```python
from build123d import *

# Parameters (mm, degrees)
ENL_V_MAT_EXTRU_1_DEPTH = 149.219431924
ESQUISSE3_R             = 3.75
ENL_V_MAT_EXTRU_2_DEPTH = 131.858702424
ENL_V_MAT_EXTRU_3_DEPTH = 126.862394907


with BuildPart() as part:
    # Esquisse1 → Révolution1 (revolve)
    with BuildSketch(Plane.XY, mode=Mode.PRIVATE) as r_volution1_sk:
        with BuildLine():
            Line((0, 0), (24.566275292, 0))
            Line((24.566275292, 0), (24.566275292, 25))
            Line((24.566275292, 25), (7.566275292, 25))
            ThreePointArc((7.566275292, 25), (6.152061729, 25.585786438), (5.566275292, 27))
            Line((5.566275292, 27), (5.566275292, 40))
            Line((5.566275292, 40), (-22.933724708, 40))
            Line((-22.933724708, 40), (-25.433724708, 37.5))
            Line((-25.433724708, 37.5), (-62.433724708, 37.5))
            Line((-62.433724708, 37.5), (-64.933724708, 40))
            Line((-64.933724708, 40), (-93.433724708, 40))
            Line((-93.433724708, 40), (-93.433724708, 27))
            ThreePointArc((-93.433724708, 27), (-94.019511146, 25.585786438), (-95.433724708, 25))
            Line((-95.433724708, 25), (-112.433724708, 25))
            Line((-112.433724708, 25), (-112.433724708, 0))
            Line((-112.433724708, 0), (0, 0))
        make_face()
    revolve(r_volution1_sk.sketch.rotate(Axis((-130.768922499, 0, 0), (1, 0, 0)), 90), axis=Axis((-130.768922499, 0, 0), (1, 0, 0)))

    # Esquisse2 → Enlèv. mat.-Extru.1 (cut, through all)
    with BuildSketch(Plane.ZY.offset(112.433724708)):
        with BuildLine():
            Line((0, 7), (0, 0))
            Line((0, 0), (43.449782835, 0))
            Line((43.449782835, 0), (43.449782835, 44.497429883))
            Line((43.449782835, 44.497429883), (0, 44.497429883))
            Line((0, 44.497429883), (0, 13))
            ThreePointArc((0, 13), (3, 10), (0, 7))
        make_face()
        with BuildLine():
            Line((-12, 7), (0, 7))
            ThreePointArc((0, 7), (3, 10), (0, 13))
            Line((0, 13), (-12, 13))
            ThreePointArc((-12, 13), (-15, 10), (-12, 7))
        make_face()
    extrude(amount=-ENL_V_MAT_EXTRU_1_DEPTH, mode=Mode.SUBTRACT)

    # Esquisse3 → Enlèv. mat.-Extru.2 (cut, through all)
    with BuildSketch(Plane.ZY.offset(93.433724708)):
        with Locations((-8.282209443, 30.909626441)):
            Circle(ESQUISSE3_R)
        with Locations((-22.627416998, 22.627416998)):
            Circle(ESQUISSE3_R)
        with Locations((-30.909626441, 8.282209443)):
            Circle(ESQUISSE3_R)
        with Locations((-30.909626441, -8.282209443)):
            Circle(ESQUISSE3_R)
        with Locations((-22.627416998, -22.627416998)):
            Circle(ESQUISSE3_R)
        with Locations((-8.282209443, -30.909626441)):
            Circle(ESQUISSE3_R)
        with Locations((8.282209443, -30.909626441)):
            Circle(ESQUISSE3_R)
        with Locations((22.627416998, -22.627416998)):
            Circle(ESQUISSE3_R)
        with Locations((30.909626441, -8.282209443)):
            Circle(ESQUISSE3_R)
    extrude(amount=-ENL_V_MAT_EXTRU_2_DEPTH, mode=Mode.SUBTRACT)

    # Esquisse4 → Enlèv. mat.-Extru.3 (cut, through all)
    with BuildSketch(Plane(origin=(0, 0, 0), x_dir=(1, 0, 0), z_dir=(0, 1, 0))):
        with BuildLine():
            Line((5.566275292, -31.140154495), (24.566275292, -40))
            Line((24.566275292, -40), (21.921370581, -25))
            Line((21.921370581, -25), (7.566275292, -25))
            ThreePointArc((7.566275292, -25), (6.152061729, -25.585786438), (5.566275292, -27))
            Line((5.566275292, -27), (5.566275292, -31.140154495))
        make_face()
        with BuildLine():
            Line((-5.433724708, -40), (5.566275292, -40))
            Line((5.566275292, -40), (5.566275292, -31.140154495))
            Line((5.566275292, -31.140154495), (-2.622958319, -27.321452148))
            ThreePointArc((-2.622958319, -27.321452148), (-4.722604922, -33.506811582), (-5.433724708, -40))
        make_face()
        with BuildLine():
            Line((-2.622958319, -27.321452148), (5.566275292, -31.140154495))
            Line((5.566275292, -31.140154495), (5.566275292, -27))
            ThreePointArc((5.566275292, -27), (6.152061729, -25.585786438), (7.566275292, -25))
            Line((7.566275292, -25), (21.921370581, -25))
            Line((21.921370581, -25), (19.356829962, -10.45576741))
            ThreePointArc((19.356829962, -10.45576741), (6.303432421, -16.199399791), (-2.622958319, -27.321452148))
        make_face()
        Polygon((5.566275292, -40), (24.566275292, -40), (5.566275292, -31.140154495), align=None)
        with BuildLine():
            Line((-7.154497255, -25.208360839), (-2.622958319, -27.321452148))
            ThreePointArc((-2.622958319, -27.321452148), (6.303432421, -16.199399791), (19.356829962, -10.45576741))
            Line((19.356829962, -10.45576741), (18.488589073, -5.531728645))
            ThreePointArc((18.488589073, -5.531728645), (3.259625276, -12.23263309), (-7.154497255, -25.208360839))
        make_face()
        with BuildLine():
            Line((21.921370581, -25), (24.566275292, -25))
            Line((24.566275292, -25), (24.566275292, -10))
            ThreePointArc((24.566275292, -10), (21.951603009, -10.114159057), (19.356829962, -10.45576741))
            Line((19.356829962, -10.45576741), (21.921370581, -25))
        make_face()
        Polygon((21.921370581, -25), (24.566275292, -40), (24.566275292, -25), align=None)
    extrude(amount=-ENL_V_MAT_EXTRU_3_DEPTH, mode=Mode.SUBTRACT)


solid = part.part
```
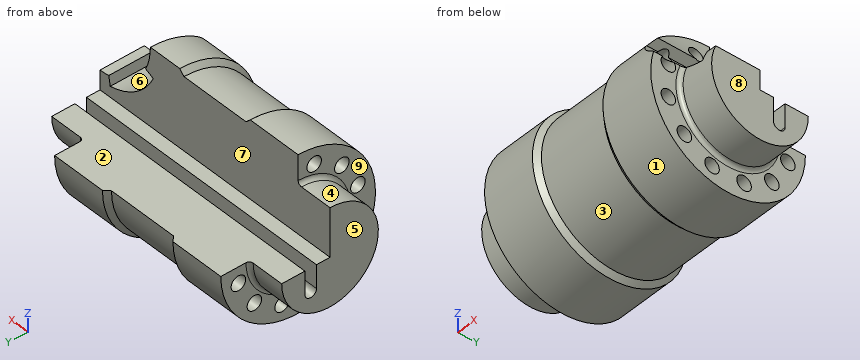
Geometry check sheet. Reference: the model listing, model coordinates, mm. Face numbers are marked on the shaded views. A direction names the side the tool comes from. Round coordinates to 2 decimals unless told otherwise and drop trailing zeros. Loops run counter-clockwise (first coordinate to the right, second up) from the corner with the lowest first, then second, coordinate; pieces in that order, holes last. Notation, with made-up numbers: (13, 28) - (37, 28) arc R21 ccw to (37, 54) - close; hole circle Ø8 at (26.5, 86). An arc over 180 degrees is marked (long way). Write each question's results on one line, items separated by ' | '. Start each with the question number.
Q1. Gauge pin test, flat ends, axial feed: P1, Ø2, axis at x = -66.5, y = 5, coming from the +Z side; P2, Ø3, axis at x = -75.5, z = -26.5, coming from the -Y side (3 decimals); P3, Ø1.5, axis at x = -92.5, z = 19, coming from the +Y side. Record the tip position at first contact, or that the pin passes through.
Q2. Thickness scan on line 1 (Y direction, x = -9, z = -26); line 2 (Y direction, x = -82, z = -7); line 3 (Y direction, x = -32, z = -7). Record the ranges inside material, lowest first. Write a range as [from, to].
Q3. Release check for a two-part mould opening along X. For the marked faces 6, 7, 8 and 9 record: +X half, -X half, draft (parallel to the pull), parting line (faces both ways), or undercut.
Q4. Cross-section at B-B on x = 1. Enter the section's corners in (y, z).
Q5. Access from +Z, -Z, +X, -X, +Y, -Y to the whole of each face (thin tool, end or side, straight path). Record for the marked faces 1, 2, 3, 4 and 5.
Q6. Cross-section at A-A on x = -44.5. State how many separate pieces and enclosed holes the cut face has, and give its area (3 significant figures).
Answers below:
1) P1: stops at z = 0 | P2: stops at y = -31.225 | P3: stops at y = 0
2) line 1: y = [-30.4, -24.27], [-20.99, 20.99], [24.27, 30.4] | line 2: y = [-39.38, -34.43], [-27.39, 7], [13, 27.39], [34.43, 39.38] | line 3: y = [-36.84, -34.43], [-27.39, 7], [13, 27.39], [34.43, 36.84]
3) face 6: undercut | face 7: draft | face 8: +X half | face 9: -X half
4) outline: (-37.42, 14.12) arc R40 ccw (long way) to (40, 0) - (13, 0) - (13, -12) arc R3 cw to (7, -12) - (7, 0) - (0, 0) - (0, 14.12) - close; hole circle Ø7.5 at (-30.91, -8.28); hole circle Ø7.5 at (-30.91, 8.28); hole circle Ø7.5 at (-22.63, -22.63); hole circle Ø7.5 at (-8.28, -30.91); hole circle Ø7.5 at (8.28, -30.91); hole circle Ø7.5 at (22.63, -22.63); hole circle Ø7.5 at (30.91, -8.28)
5) face 1: +X, -X | face 2: +Z, +X, -X, +Y | face 3: none | face 4: -X | face 5: +Z, -Z, -X, +Y, -Y
6) separate pieces: 1 | enclosed holes: 9 | area: 2,830 mm²
